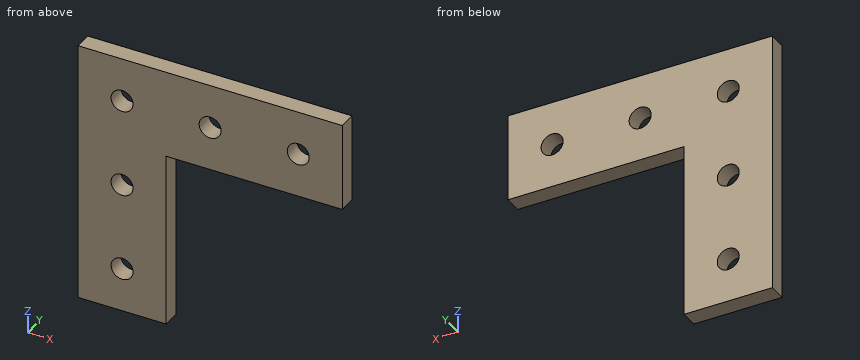
```python
from build123d import *

# Parameters (mm, degrees)
BOSS_EXTRUDE1_DEPTH             = 5.08
F_1_4_0_25_DIAMETER_HOLE1_D     = 6.35
F_1_4_0_25_DIAMETER_HOLE1_DEPTH = 25.4
F_1_4_0_25_DIAMETER_HOLE1_TIP   = 1.907732465


with BuildPart() as part:
    # Sketch1 → Boss-Extrude1 (new body)
    with BuildSketch(Plane(origin=(0, 0, 0), x_dir=(1, 0, 0), z_dir=(0, 1, 0))):
        Polygon((0, 0), (0, 76.2), (25.4, 76.2), (25.4, 25.4), (76.2, 25.4), (76.2, 0), align=None)
    extrude(amount=BOSS_EXTRUDE1_DEPTH)

    # 1/4 (0.25) Diameter Hole1
    with Locations(Plane(origin=(0, 5.08, 0), x_dir=(1, 0, 0), z_dir=(0, 1, 0))):
        with Locations((12.7, 63.5), (12.7, 38.1), (12.7, 12.7), (38.1, 12.7), (63.5, 12.7)):
            Hole(F_1_4_0_25_DIAMETER_HOLE1_D / 2, depth=F_1_4_0_25_DIAMETER_HOLE1_DEPTH)
            with Locations((0, 0, -(F_1_4_0_25_DIAMETER_HOLE1_DEPTH + F_1_4_0_25_DIAMETER_HOLE1_TIP / 2))):  # 118° drill point
                Cone(0, F_1_4_0_25_DIAMETER_HOLE1_D / 2, F_1_4_0_25_DIAMETER_HOLE1_TIP, mode=Mode.SUBTRACT)


solid = part.part
```
Geometry: final body of the model. Coordinates: model frame, mm. Give positions to 0.01 mm unless a question says otherwise; leave off trailing zeros. Write each loop counter-clockwise with the first axis right and the second up, starting at its lowest first coordinate (ties: lowest second). Pieces come first, ordered by that corner, then holes.
1. Pin query (flat end, axial travel): P1, Ø1, axis at x = 53, y = 2.5, coming from the -Z side; P2, Ø2.5, axis at y = 3.5, z = -55.5, coming from the +X side. Return the tip coordinate at first contact, or that it passes through.
2. Section query D-D, the plane x = 63.5. Return loops of the section in (y, z) (3 decimals).
3. Section query C-C, the plane y = 3.2. Return loops of the section in (x, z) (3 decimals).
4. Line query: probe 1 along X at (y, z) = (2.15, -12.7) (3 decimals); probe 2 along Z at (x, y) = (12.7, 3.65) (3 decimals); probe 3 along Z at (x, y) = (38.1, 3.55) (3 decimals). Output: solid intervals per line, ascending.
5. Section query B-B, the plane z = -12.7. Return loops of the section in (x, y) (3 decimals).
6. Section query A-A, the plane x = 12.7. Return loops of the section in (y, z) (3 decimals), then the cut area to 3 significant figures.
Computed:
1. P1: stops at z = -25.4
1. P2: stops at x = 25.4
2. outline: (0, -25.4) - (5.08, -25.4) - (5.08, -15.875) - (0, -15.875) - close; (0, -9.525) - (5.08, -9.525) - (5.08, 0) - (0, 0) - close
3. outline: (0, -76.2) - (25.4, -76.2) - (25.4, -25.4) - (76.2, -25.4) - (76.2, 0) - (0, 0) - close; hole circle Ø6.35 at (12.7, -63.5); hole circle Ø6.35 at (12.7, -38.1); hole circle Ø6.35 at (12.7, -12.7); hole circle Ø6.35 at (38.1, -12.7); hole circle Ø6.35 at (63.5, -12.7)
4. probe 1: x = 0 to 9.525, 15.875 to 34.925, 41.275 to 60.325, 66.675 to 76.2
4. probe 2: z = -76.2 to -66.675, -60.325 to -41.275, -34.925 to -15.875, -9.525 to 0
4. probe 3: z = -25.4 to -15.875, -9.525 to 0
5. outline: (0, 0) - (9.525, 0) - (9.525, 5.08) - (0, 5.08) - close; (15.875, 0) - (34.925, 0) - (34.925, 5.08) - (15.875, 5.08) - close; (41.275, 0) - (60.325, 0) - (60.325, 5.08) - (41.275, 5.08) - close; (66.675, 0) - (76.2, 0) - (76.2, 5.08) - (66.675, 5.08) - close
6. outline: (0, -76.2) - (5.08, -76.2) - (5.08, -66.675) - (0, -66.675) - close; (0, -60.325) - (5.08, -60.325) - (5.08, -41.275) - (0, -41.275) - close; (0, -34.925) - (5.08, -34.925) - (5.08, -15.875) - (0, -15.875) - close; (0, -9.525) - (5.08, -9.525) - (5.08, 0) - (0, 0) - close
6. area: 290 mm2
